Check sheet for the modelled part. Datum: model origin and axes. Units: mm. Face numbers are marked on the shaded views. A direction names the side the tool comes from. Round coordinates to 2 decimals unless told otherwise and drop trailing zeros. Loops run counter-clockwise (first coordinate to the right, second up) from the corner with the lowest first, then second, coordinate; pieces in that order, holes last. Notation, with made-up numbers: (-28.75, 76) - (17.25, 76) arc R11 cw to (17.25, 88) - close; hole circle Ø9 at (56.25, 70). An arc over 180 degrees is marked (long way). Answer in a Markdown table with one row per item. Add a question column.
(1) Cross-section at A-A on x = 0. Enter the section's corners in (y, z).
(2) Cross-section at D-D on y = -2.75. Enter the section's corners in (x, z), then the cut area to 3 significant figures.
(3) Gauge pin test, flat ends, axial feed: pin 1 (6.5 mm diameter, centred on x = 0, z = 0, fed in from -Y); pin 2 (6 mm diameter, centred on y = 0, z = 15, fed in from -X); pin 3 (1.5 mm diameter, centred on x = -13, y = 2, fed in from +Z). Record the tip position at first contact, or that the pin passes through.
(4) Thickness scan on line 1 along X through (y, z) = (1.55, 0); line 2 along Y through (x, z) = (-17.5, 22.5). Record the ranges inside material, lowest first.
(5) Access from +Z, -Z, +X, -X, +Y, -Y to the whole of each face (thin tool, end or side, straight path). Record for the marked faces 1 and 2.
(6) Cross-section at C-C on y = 2.75. Enter the section's corners in (x, z), then the cut area to 3 significant figures.
(7) Cross-section at B-B on z = 0. Enter the section's corners in (x, y).
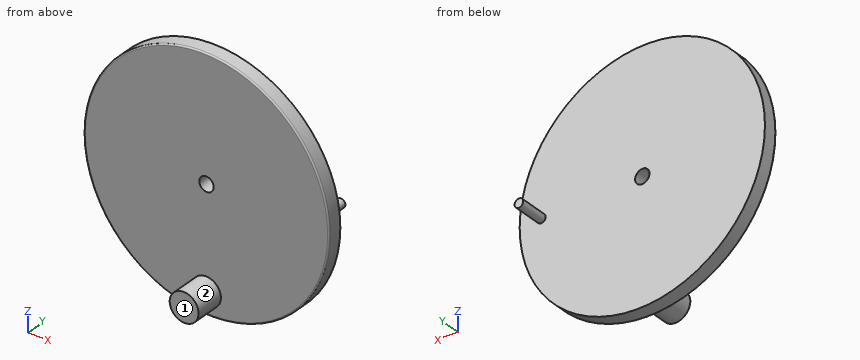
from build123d import *

# Parameters (mm, degrees)
SKETCH1_R           = 42.5
BOSS_EXTRUDE1_DEPTH = 5
SKETCH2_R           = 1.5
BOSS_EXTRUDE2_DEPTH = 10
SKETCH3_R           = 2.5
CUT_EXTRUDE1_DEPTH  = 10
SKETCH4_R           = 5
BOSS_EXTRUDE3_DEPTH = 10
FILLET1_R           = 0.5


with BuildPart() as part:
    # Sketch1 → Boss-Extrude1 (new body)
    with BuildSketch(Plane(origin=(0, 0, 0), x_dir=(1, 0, 0), z_dir=(0, 1, 0))):
        Circle(SKETCH1_R)
    extrude(amount=BOSS_EXTRUDE1_DEPTH)

    # Sketch2 → Boss-Extrude2 (add)
    with BuildSketch(Plane(origin=(0, 5, 0), x_dir=(1, 0, 0), z_dir=(0, 1, 0))):
        with Locations((35, 0)):
            Circle(SKETCH2_R)
    extrude(amount=BOSS_EXTRUDE2_DEPTH)

    # Sketch3 → Cut-Extrude1 (cut)
    with BuildSketch(Plane(origin=(0, 5, 0), x_dir=(1, 0, 0), z_dir=(0, 1, 0))):
        Circle(SKETCH3_R)
    extrude(amount=-CUT_EXTRUDE1_DEPTH, mode=Mode.SUBTRACT)

    # Sketch4 → Boss-Extrude3 (add)
    with BuildSketch(Plane.XZ):
        with Locations((0, -35)):
            Circle(SKETCH4_R)
    extrude(amount=BOSS_EXTRUDE3_DEPTH)

    # Fillet1
    fillet1_edges = [part.edges().sort_by_distance(p)[0] for p in [
        (-42.5, 0, 0),
    ]]
    fillet(fillet1_edges, radius=FILLET1_R)


solid = part.part
Answers:
| question | item | result |
|---|---|---|
| 1 | outline | (-10, -40) - (0, -40) - (0, -42) arc R0.5 ccw to (0.5, -42.5) - (5, -42.5) - (5, -2.5) - (0, -2.5) - (0, -30) - (-10, -30) - close; (0, 2.5) - (5, 2.5) - (5, 42.5) - (0.5, 42.5) arc R0.5 ccw to (0, 42) - close |
| 2 | outline | circle Ø10 at (0, -35) |
| 2 | area | 78.5 mm^2 |
| 3 | pin 1 | stops at y = 0 |
| 3 | pin 2 | stops at x = -40.76 |
| 3 | pin 3 | stops at z = 40.7 |
| 4 | line 1 | x = -42.5 to -2.5, 2.5 to 42.5 |
| 4 | line 2 | y = 0 to 5 |
| 5 | face 1 | +Z, -Z, +X, -X, -Y |
| 5 | face 2 | -Y |
| 6 | outline | circle Ø85 at (0, 0); hole circle Ø5 at (0, 0) |
| 6 | area | 5,650 mm^2 |
| 7 | outline | (-42.5, 0.5) arc R0.5 ccw to (-42, 0) - (-2.5, 0) - (-2.5, 5) - (-42.5, 5) - close; (2.5, 0) - (42, 0) arc R0.5 ccw to (42.5, 0.5) - (42.5, 5) - (36.5, 5) - (36.5, 15) - (33.5, 15) - (33.5, 5) - (2.5, 5) - close |
